Read the model definition and answer for the solid it produces. Units are mm, in the model's axes. Round coordinates to 2 decimals unless told otherwise and drop trailing zeros. Order: outer loops, then holes, each group sorted by start corner. A loop starts at its lowest first (then second) coordinate and runs counter-clockwise, first axis right, second up. Notation, with made-up numbers: M 72,12 L 81,12 A26 cw 81,33 Z; hole C 45.25,-36 d4. An arc over 180 degrees is marked long. Answer as CSV lines item,"result".
```python
from build123d import *

# Parameters (mm, degrees)
F0_R     = 5.55625
F1_DEPTH = 6.35


with BuildPart() as f1:
    # F0 (on Top) → F1 (new body)
    with BuildSketch(Plane.XY):
        with BuildLine():
            Line((0, 50.8), (0, 0))
            Line((0, 0), (609.6, 0))
            Line((609.6, 0), (609.6, 50.8))
            Line((609.6, 50.8), (533.4, 127))
            Line((533.4, 127), (438.246727, 127))
            ThreePointArc((438.246727, 127), (304.8, 49.53), (171.353273, 127))
            Line((171.353273, 127), (76.2, 127))
            Line((76.2, 127), (0, 50.8))
        make_face()
        with Locations((304.8, 36.5125)):
            Circle(F0_R, mode=Mode.SUBTRACT)
        with Locations((186.934138, 85.334138)):
            Circle(F0_R, mode=Mode.SUBTRACT)
        with Locations((422.665862, 85.334138)):
            Circle(F0_R, mode=Mode.SUBTRACT)
    extrude(amount=F1_DEPTH)


solid = f1.part
```
Item 1: Determine the mould class of faces 1 (the face through (38.6, 89.4, 3.1)), 2 (the face through (182.84, 89.09, 3.13)), 3 (the face through (301, 22, 0)), 4 (the face through (299.25, 36.76, 3.13)) for opening direction Y: +Y half, -Y half, draft (parallel to the pull), parting line (faces both ways), or undercut.
Ans:
face 1,"+Y half"
face 2,"undercut"
face 3,"draft"
face 4,"undercut"
Item 2: A flat-ended cylindrical pin translates along its axis: pin 1 (1.5 mm diameter, centred on y = 85, z = 1.5, fed in from -X). Find the tip coordinate at first contact, or state that the pin passes through.
Ans:
pin 1,"x = 33.45"
Item 3: Find the intervals of material crossed by probe 1 along X at (y, z) = (86, 1.5); probe 2 along Y at (x, z) = (304.8, 3); probe 3 along X at (y, z) = (61, 4.25), in increasing order. Write a range as [from, to].
Ans:
probe 1,"[35.2, 181.42], [192.45, 205.41], [404.19, 417.15], [428.18, 574.4]"
probe 2,"[0, 30.96], [42.07, 49.53]"
probe 3,"[10.2, 246.55], [363.05, 599.4]"
Item 4: A cutting plane is placed at C-C, the plane z = 1.25. Determine the outline of the cut face in (x, y).
Ans:
outline,"M 0,0 L 609.6,0 L 609.6,50.8 L 533.4,127 L 438.25,127 A153.67 cw 171.35,127 L 76.2,127 L 0,50.8 Z; hole C 186.93,85.33 d11.11; hole C 304.8,36.51 d11.11; hole C 422.67,85.33 d11.11"
Item 5: A cutting plane is placed at A-A, the plane x = 304.8. Determine the outline of the cut face in (y, z), and give its area (3 significant figures).
Ans:
outline,"M 0,0 L 30.96,0 L 30.96,6.35 L 0,6.35 Z; M 42.07,0 L 49.53,0 L 49.53,6.35 L 42.07,6.35 Z"
area,"244 mm2"
Item 6: A cutting plane is placed at B-B, the plane y = 69.5. Determine the outline of the cut face in (x, z).
Ans:
outline,"M 18.7,0 L 229.05,0 L 229.05,6.35 L 18.7,6.35 Z; M 380.55,0 L 590.9,0 L 590.9,6.35 L 380.55,6.35 Z"
Item 7: A cutting plane is placed at D-D, the plane x = 208. Determine the outline of the cut face in (y, z), and give its area (3 significant figures).
Ans:
outline,"M 0,0 L 83.85,0 L 83.85,6.35 L 0,6.35 Z"
area,"532 mm2"
